Geometry check sheet. Reference: the model listing, model coordinates, mm. A direction names the side the tool comes from. Round coordinates to 2 decimals unless told otherwise and drop trailing zeros. Order: outer loops, then holes, each group sorted by start corner. A loop starts at its lowest first (then second) coordinate and runs counter-clockwise, first axis right, second up. Notation, with made-up numbers: (2, -24) - (37, -24) arc R20 cw to (37, 6) - close; hole circle Ø11 at (-3.5, 41). An arc over 180 degrees is marked (long way). Write each question's results on one line, items separated by ' | '.
```python
from build123d import *

# Parameters (mm, degrees)
BOSS_EXTRUDE1_DEPTH      = 7.62
BOSS_EXTRUDE2_DEPTH      = 12.7
BOSS_EXTRUDE2_DEPTH_BACK = 25.4
SKETCH2_W                = 7.62
SKETCH2_H                = 25.4
SKETCH3_W                = 19.05
SKETCH3_H                = 7.62
CUT_EXTRUDE1_DEPTH       = 182.02289717


with BuildPart() as part:
    # Sketch1 → Boss-Extrude1 (new body)
    with BuildSketch(Plane.XY):
        Polygon((0, 0), (12.7, 0), (12.7, 165.1), (25.4, 165.1), (25.4, 171.45), (12.7, 171.45), (12.7, 179.07), (0, 179.07), (0, 171.45), (-12.7, 171.45), (-12.7, 165.1), (0, 165.1), align=None)
    extrude(amount=BOSS_EXTRUDE1_DEPTH)

    # Sketch2 → Boss-Extrude2 (add, two sides: drawn at the far end of the back side and taken through both)
    with BuildSketch(Plane.ZY.offset(-BOSS_EXTRUDE2_DEPTH_BACK)):
        with Locations((3.81, 38.1)):
            Rectangle(SKETCH2_W, SKETCH2_H)
    extrude(amount=BOSS_EXTRUDE2_DEPTH + BOSS_EXTRUDE2_DEPTH_BACK)

    # Sketch3 → Cut-Extrude1 (cut, through all)
    with BuildSketch(Plane.XY.offset(7.62)):
        with Locations((6.35, 38.1)):
            Rectangle(SKETCH3_W, SKETCH3_H)
    extrude(amount=-CUT_EXTRUDE1_DEPTH, mode=Mode.SUBTRACT)


solid = part.part
```
(1) Depth check by flat-ended pin: pin 1 Ø2.5 at (y, z) = (174, 2.5) entering from -X; pin 2 Ø2.5 at (x, z) = (17.5, 2.5) entering from +Y; pin 3 Ø4 at (x, z) = (-4.5, 2.5) entering from -Y. Enter the tip coordinate at first touch or a pass-through.
Answers follow:
pin 1: x = 0 | pin 2: y = 171.45 | pin 3: y = 25.4
(2) Material ranges on line 1 (Y direction, x = 13.5, z = 4.5); line 2 (Y direction, x = 2.5, z = 7); line 3 (X direction, y = 35.5, z = 5) (3 decimals), recorded low to high.
Answers follow:
line 1: 25.4 to 34.29, 41.91 to 50.8, 165.1 to 171.45 | line 2: 0 to 34.29, 41.91 to 179.07 | line 3: -12.7 to -3.175, 15.875 to 25.4
(3) Section check A-A (x = -9). Record the cut outline in (y, z), then the cut area to 3 significant figures.
Answers follow:
outline: (25.4, 0) - (50.8, 0) - (50.8, 7.62) - (25.4, 7.62) - close; (165.1, 0) - (171.45, 0) - (171.45, 7.62) - (165.1, 7.62) - close | area: 242 mm²
(4) Draft check along X on faces 4 (the face through (15.875, 38, 4)), 5 (the face through (19, 50.8, 4)), 6 (the face through (0, 175, 4)), 7 (the face through (-3.175, 38, 4)). Enter one of: released by +X, released by -X, zero draft, split by the parting line, or undercut.
Answers follow:
face 4: undercut | face 5: zero draft | face 6: released by -X | face 7: undercut
(5) Section check B-B (x = -1.5). Record the cut outline in (y, z), then the cut area to 3 significant figures.
Answers follow:
outline: (25.4, 0) - (34.29, 0) - (34.29, 7.62) - (25.4, 7.62) - close; (41.91, 0) - (50.8, 0) - (50.8, 7.62) - (41.91, 7.62) - close; (165.1, 0) - (171.45, 0) - (171.45, 7.62) - (165.1, 7.62) - close | area: 184 mm²
(6) Access from +Z, -Z, +X, -X, +Y, -Y to the whole of each face (thin tool, end or side, straight path). Record for faces 1 (the face through (19, 165.1, 4)), 2 (the face through (0, 109, 4)), 3 (the face through (12.7, 175, 4)).
Answers follow:
face 1: +Z, -Z, +X | face 2: +Z, -Z, -X | face 3: +Z, -Z, +X, +Y
(7) Section check C-C (z = 2). Record the cut outline in (x, y) (3 decimals).
Answers follow:
outline: (-12.7, 25.4) - (0, 25.4) - (0, 0) - (12.7, 0) - (12.7, 25.4) - (25.4, 25.4) - (25.4, 50.8) - (12.7, 50.8) - (12.7, 165.1) - (25.4, 165.1) - (25.4, 171.45) - (12.7, 171.45) - (12.7, 179.07) - (0, 179.07) - (0, 171.45) - (-12.7, 171.45) - (-12.7, 165.1) - (0, 165.1) - (0, 50.8) - (-12.7, 50.8) - close; hole (-3.175, 34.29) - (15.875, 34.29) - (15.875, 41.91) - (-3.175, 41.91) - close
(8) Section check D-D (y = 75). Record the cut outline in (x, z).
Answers follow:
outline: (0, 0) - (12.7, 0) - (12.7, 7.62) - (0, 7.62) - close
